```python
from build123d import *

# Parameters (mm, degrees)
SKETCH1_R           = 16
SKETCH1_R_2         = 13.6
BOSS_EXTRUDE1_DEPTH = 50
CUT_EXTRUDE1_DEPTH  = 55.881690936
CUT_EXTRUDE2_DEPTH  = 3.5


with BuildPart() as part:
    # Sketch1 → Boss-Extrude1 (new body)
    with BuildSketch(Plane(origin=(0, 0, 0), x_dir=(0, 0, -1), z_dir=(1, 0, 0))):
        Circle(SKETCH1_R)
        Circle(SKETCH1_R_2, mode=Mode.SUBTRACT)
    extrude(amount=BOSS_EXTRUDE1_DEPTH)

    # Sketch2 → Cut-Extrude1 (cut, through all)
    with BuildSketch(Plane(origin=(50, 0, 0), x_dir=(0, 0, -1), z_dir=(1, 0, 0))):
        with BuildLine():
            Line((-8.1, 12.743625858), (-7.295364238, 11.477702759))
            ThreePointArc((-7.295364238, 11.477702759), (0, 13.6), (7.295364238, 11.477702759))
            Line((7.295364238, 11.477702759), (8.1, 12.743625858))
            ThreePointArc((8.1, 12.743625858), (0, 15.1), (-8.1, 12.743625858))
        make_face()
        with BuildLine():
            Line((-8.1, -12.743625858), (-7.295364238, -11.477702759))
            ThreePointArc((-7.295364238, -11.477702759), (0.008056302, -13.599997614), (7.308957327, -11.469051521))
            Line((7.308957327, -11.469051521), (8.1, -12.743625858))
            ThreePointArc((8.1, -12.743625858), (0, -15.1), (-8.1, -12.743625858))
        make_face()
    extrude(amount=-CUT_EXTRUDE1_DEPTH, mode=Mode.SUBTRACT)

    # Sketch3 → Cut-Extrude2 (cut)
    with BuildSketch(Plane(origin=(0, 0, 0), x_dir=(-1, 0, 0), z_dir=(0, -0.5364238410596023, -0.8439487322953112))):
        with BuildLine():
            Line((-7, -13.6), (-7, -12.445895529))
            Line((-7, -12.445895529), (-25, -12.445895529))
            Line((-25, -12.445895529), (-25, -13.6))
            add(Edge.make_bspline(
                [(-25, -13.6), (-25.419648133, -14.53323317), (-22.215303237, -14.299464122), (-19.182889181, -14.398286796), (-18.428629005, -14.414668585), (-16.283931227, -14.396819072), (-13.186228061, -14.668811806), (-11.028088937, -13.12651294), (-8.819150609, -14.976468108), (-7, -13.6)],
                knots=[0, 0, 0, 0, 0.204097014, 0.238608821, 0.396578619, 0.439763334, 0.627271258, 0.685638773, 1, 1, 1, 1], degree=3))
        make_face()
    extrude(amount=-CUT_EXTRUDE2_DEPTH, mode=Mode.SUBTRACT)


solid = part.part
```
Can you work these out from the model? Positions are in its coordinate system, mm. A direction names the side the tool comes from. Give positions to 0.01 mm unless a question says otherwise; leave off trailing zeros. Order: outer loops, then holes, each group sorted by start corner. A loop starts at its lowest first (then second) coordinate and runs counter-clockwise, first axis right, second up. Notation, with made-up numbers: M -39.75,-12 L -16.75,-12 A20 cw -16.75,9 Z; hole C 58.25,-1.5 d4. An arc over 180 degrees is marked long. Write item = value, one per line. Start each with the question number.
Q1. Suppose I cut it at A-A (y = 0). Write out the boundary of the cut face in (x, z), plus the area to 3 significant figures.
Q2. Suppose I cut it at B-B (x = 39). Write out the boundary of the cut face in (y, z), plus the area to 3 significant figures.
Q3. We'd pull the mould along Y, two halves only. Please class faces 1 (the cylindrical face through (24.65, -15.62, 3.47)), 2 (the cylindrical face through (24.6, -0.2, -13.6)), 3 (the flat face through (50, -7, 12)): pulls with the +Y half, pulls with the -Y half, needs draft (parallel to the pull), parting line crosses it, or undercut.
Q4. I need wall thicknesses on probe 1 along Y at (x, z) = (9, -0.5); probe 2 along Z at (x, y) = (19, 4); probe 3 along Z at (x, y) = (36, -8). Which ranges of each line are inside material? Lowest first, please. Write a range as [from, to].
Q5. Will these pins go through, and if not, where does the flat tip stop? pin 1 Ø12 at (x, z) = (7, 9) entering from +Y; pin 2 Ø8 at (x, y) = (29.5, -5) entering from +Z; pin 3 Ø1 at (x, y) = (15, 3) entering from +Z.
Q6. For faces 4 (the cylindrical face through (25.4, 15.1, -0.1)), 5 (the flat face through (16.34, -9.62, 10.26)), 6 (the flat face through (0, -7, 12)), which set-ups out of +Z, -Z, +X, -X, +Y, -Y let a thin tool reach every point of the face, with its end or its side?
Q7. Suppose I cut it at C-C (z = 0). Write out the boundary of the cut face in (x, y), plus the area to 3 significant figures.
Check result:
q1.outline = M 0,-16 L 50,-16 L 50,-13.6 L 0,-13.6 Z; M 0,13.6 L 50,13.6 L 50,16 L 0,16 Z
q1.area = 240 mm2
q2.outline = C 0,0 d32; hole M -12.74,-8.1 L -11.47,-7.31 A13.6 ccw 11.48,-7.3 L 12.74,-8.1 A15.1 ccw 12.74,8.1 L 11.48,7.3 A13.6 ccw -11.48,7.3 L -12.74,8.1 A15.1 ccw Z
q2.area = 174 mm2
q3.face_1 = parting line crosses it
q3.face_2 = undercut
q3.face_3 = needs draft
q4.probe_1 = [-15.99, -15.09], [15.09, 15.99]
q4.probe_2 = [-15.49, -13], [13, 15.49]
q4.probe_3 = [-13.86, -11], [11, 13.86]
q5.pin_1 = 15.72
q5.pin_2 = 15.97
q5.pin_3 = 15.8
q6.face_4 = +X, -X
q6.face_5 = none
q6.face_6 = +Z, -Z, -X, +Y, -Y
q7.outline = M 0,-16 L 50,-16 L 50,-15.1 L 0,-15.1 Z; M 0,15.1 L 50,15.1 L 50,16 L 0,16 Z
q7.area = 90.0 mm2
